Build history of the part. All positions in model axes, mm. A direction names the side the tool comes from. Give positions to 0.01 mm unless a question says otherwise; leave off trailing zeros. Order: outer loops, then holes, each group sorted by start corner. A loop starts at its lowest first (then second) coordinate and runs counter-clockwise, first axis right, second up. Notation, with made-up numbers: (-12, 55.25) - (24, 55.25) arc R17 ccw to (24, 65.25) - close; hole circle Ø10 at (-20, -36.75). An arc over 180 degrees is marked (long way). Answer in a Markdown table with one row per item.
```python
from build123d import *

# Parameters (mm, degrees)
EXTRUDE_1_DEPTH             = 16
CUT_EXTRUDE_1_DEPTH         = 13
CUT_EXTRUDE_2_DEPTH         = 17
CUT_EXTRUDE_3_DEPTH         = 17
HOLE_WIZARD_1_5_1_5_1_D     = 1.5
HOLE_WIZARD_1_5_1_5_1_DEPTH = 35.5
HOLE_WIZARD_12_0_12_1_D     = 12
HOLE_WIZARD_12_0_12_1_DEPTH = 16
HOLE_WIZARD_3_6_3_6_1_D     = 3.6
HOLE_WIZARD_3_6_3_6_1_DEPTH = 16
FILLET_1_R                  = 2
FILLET_2_R                  = 3


with BuildPart() as part:
    # 草图1 → 凸台-拉伸1 (new body)
    with BuildSketch(Plane(origin=(0, 0, 0), x_dir=(-1, 0, 0), z_dir=(0, 0, -1))):
        with BuildLine():
            Line((442.70274024, 283), (457.29725976, 283))
            ThreePointArc((457.29725976, 283), (450, 318.5), (442.70274024, 283))
        make_face()
    extrude(amount=-EXTRUDE_1_DEPTH)

    # 草图2 → 切除-拉伸1 (cut)
    with BuildSketch(Plane.XY.offset(16)):
        with BuildLine():
            Line((-461.891570779, 285.828177802), (-460.908295205, 287))
            Line((-460.908295205, 287), (-439.091704795, 287))
            Line((-439.091704795, 287), (-438.108429221, 285.828177802))
            ThreePointArc((-438.108429221, 285.828177802), (-450, 318.5), (-461.891570779, 285.828177802))
        make_face()
    extrude(amount=-CUT_EXTRUDE_1_DEPTH, mode=Mode.SUBTRACT)

    # 草图3 → 切除-拉伸2 (cut, through all)
    with BuildSketch(Plane(origin=(0, 0, 0), x_dir=(-1, 0, 0), z_dir=(0, 0, -1))):
        with BuildLine():
            Line((431.781056569, 296.787508713), (435.227883705, 297.395277335))
            ThreePointArc((435.227883705, 297.395277335), (437.009618943, 307.5), (444.86969785, 314.095389312))
            Line((444.86969785, 314.095389312), (443.672627348, 317.384313485))
            ThreePointArc((443.672627348, 317.384313485), (433.97853003, 309.25), (431.781056569, 296.787508713))
        make_face()
    extrude(amount=-CUT_EXTRUDE_2_DEPTH, mode=Mode.SUBTRACT)

    # 草图4 → 切除-拉伸3 (cut, through all)
    with BuildSketch(Plane(origin=(0, 0, 0), x_dir=(-1, 0, 0), z_dir=(0, 0, -1))):
        with BuildLine():
            Line((456.327372652, 317.384313485), (455.13030215, 314.095389312))
            ThreePointArc((455.13030215, 314.095389312), (462.990381057, 307.5), (464.772116295, 297.395277335))
            Line((464.772116295, 297.395277335), (468.218943431, 296.787508713))
            ThreePointArc((468.218943431, 296.787508713), (466.02146997, 309.25), (456.327372652, 317.384313485))
        make_face()
    extrude(amount=-CUT_EXTRUDE_3_DEPTH, mode=Mode.SUBTRACT)

    # Ø1.5 (1.5) 直径孔1
    with Locations(Plane(origin=(0, 283, 0), x_dir=(-1, 0, 0), z_dir=(0, -1, 0))):
        with Locations((446.75, -11), (453.25, -11)):
            Hole(HOLE_WIZARD_1_5_1_5_1_D / 2, depth=HOLE_WIZARD_1_5_1_5_1_DEPTH)

    # Ø12.0 (12) 直径孔1
    with Locations(Plane(origin=(0, 0, 0), x_dir=(-1, 0, 0), z_dir=(0, 0, -1))):
        with Locations((450, 300)):
            Hole(HOLE_WIZARD_12_0_12_1_D / 2, depth=HOLE_WIZARD_12_0_12_1_DEPTH)

    # Ø3.6 (3.6) 直径孔1
    with Locations(Plane(origin=(0, 0, 0), x_dir=(-1, 0, 0), z_dir=(0, 0, -1))):
        with Locations((437.009618943, 292.5), (450, 315), (462.990381057, 292.5)):
            Hole(HOLE_WIZARD_3_6_3_6_1_D / 2, depth=HOLE_WIZARD_3_6_3_6_1_DEPTH)

    # 圆角1
    fillet_1_edges = [part.edges().sort_by_distance(p)[0] for p in [
        (-444.86969785, 314.095389312, 1.5),
        (-435.227883705, 297.395277335, 1.5),
        (-464.772116295, 297.395277335, 1.5),
        (-455.13030215, 314.095389312, 1.5),
    ]]
    fillet(fillet_1_edges, radius=FILLET_1_R)

    # 圆角2
    fillet_2_edges = [part.edges().sort_by_distance(p)[0] for p in [
        (-438.600067008, 286.414088901, 3),
        (-450, 287, 3),
        (-461.399932992, 286.414088901, 3),
    ]]
    fillet(fillet_2_edges, radius=FILLET_2_R)


solid = part.part
```
1. Drop flat-ended pins along their axis: P1, Ø9, axis at x = -449.5, y = 308.5, coming from the +Z side; P2, Ø1, axis at x = -441.5, z = 5.5, coming from the -Y side; P3, Ø3, axis at x = -447, z = 12.5, coming from the +Y side; P4, Ø4, axis at x = -435.5, z = 14, coming from the +Y side (3 decimals). Give the stop position or say it passes through.
Check result:
| item | result |
|---|---|
| P1 | stops at z = 3 |
| P2 | stops at y = 283.32 |
| P3 | stops at y = 287 |
| P4 | passes through |
2. Cut at B-B on z = 11. Write the cut outline in (x, y), and give its area (3 significant figures).
Check result:
| item | result |
|---|---|
| outline | (-461.89, 285.83) arc R18.5 ccw to (-457.3, 283) - (-454, 283) - (-454, 287) - (-460.91, 287) - close; (-452.5, 283) - (-447.5, 283) - (-447.5, 287) - (-452.5, 287) - close; (-446, 283) - (-442.7, 283) arc R18.5 ccw to (-438.11, 285.83) - (-439.09, 287) - (-446, 287) - close |
| area | 70.4 mm² |
3. Which spindle directions (+Z, -Z, +X, -X, +Y, -Y) get a long thin tool onto all of the face, cutting with end or side? Do faces 4 (the face through (-450, 283, 8)), 5 (the face through (-438.607, 286.422, 11.07)), 6 (the face through (-456.055, 316.635, 1.479)). Say none if no direction does.
Check result:
| item | result |
|---|---|
| face 4 | +Z, -Z, +X, -X, -Y |
| face 5 | +Z, +X, +Y |
| face 6 | +Z, -Z, -X |
4. Cut at A-A on x = -450. Write the cut outline in (y, z), and give its area (3 significant figures).
Check result:
| item | result |
|---|---|
| outline | (283, 0) - (294, 0) - (294, 3) - (290, 3) arc R3 cw to (287, 6) - (287, 16) - (283, 16) - close; (306, 0) - (313.2, 0) - (313.2, 3) - (306, 3) - close; (316.8, 0) - (318.5, 0) - (318.5, 3) - (316.8, 3) - close |
| area | 114 mm² |
5. Cut at D-D on z = 14.5. Write the cut outline in (x, y), and give its area (3 significant figures).
Check result:
| item | result |
|---|---|
| outline | (-461.89, 285.83) arc R18.5 ccw to (-457.3, 283) - (-442.7, 283) arc R18.5 ccw to (-438.11, 285.83) - (-439.09, 287) - (-460.91, 287) - close |
| area | 82.4 mm² |
6. Cut at C-C on y = 315. Write the cut outline in (x, z), and give its area (3 significant figures).
Check result:
| item | result |
|---|---|
| outline | (-455.66, 0) - (-451.8, 0) - (-451.8, 3) - (-455.66, 3) - close; (-448.2, 0) - (-444.34, 0) - (-444.34, 3) - (-448.2, 3) - close |
| area | 23.2 mm² |
7. Probe line 1 (Y direction, x = -450, z = 1.65); line 2 (X direction, y = 285.2, z = 11); line 3 (X direction, y = 284.25, z = 11). List the from-to ranges inside material, lowest first.
Check result:
| item | result |
|---|---|
| line 1 | y = 283 to 294, 306 to 313.2, 316.8 to 318.5 |
| line 2 | x = -461.1 to -454, -452.5 to -447.5, -446 to -438.9 |
| line 3 | x = -459.71 to -454, -452.5 to -447.5, -446 to -440.29 |
8. Two-plate mould, pull along X, no slides. Class faces 1 (the face through (-449.83, 287.9, 3.86)), 2 (the face through (-452.535, 285.028, 10.775)), 3 (the face through (-462.15, 287.56, 3.52)): +X half, -X half, draft (parallel to the pull), parting line (faces both ways), or undercut.
Check result:
| item | result |
|---|---|
| face 1 | draft |
| face 2 | undercut |
| face 3 | -X half |
